Here's how the part is built. I have some questions about the finished solid (model axes, mm). Face numbers are marked on the shaded views. Coordinates: 2 decimals unless noted, no trailing zeros. Write each loop counter-clockwise with the first axis right and the second up, starting at its lowest first coordinate (ties: lowest second). Pieces come first, ordered by that corner, then holes.
(1) Thinking about a two-plate mould opening in Z: for the marked faces 1 and 2, which applies, released by +Z, released by -Z, zero draft, split by the parting line, or undercut?
(2) For pin 1 Ø1.5 at (x, z) = (239, -0.5) entering from +Y, with a flat end and sliding along its axis, tell me the tip position at first contact or that it passes through.
(3) Imagine slicing it at A-A, the plane x = 247. List the corners of the cut face in (y, z) for me, plus the area to 3 significant figures.
(4) Imagine slicing it at C-C, the plane x = 222. List the corners of the cut face in (y, z) for me.
(5) Imagine slicing it at B-B, the plane y = 166.5. List the corners of the cut face in (x, z) for me, plus the area to 3 significant figures.
(6) Please list where these lines run through material, in increasing order: probe 1 along X at (y, z) = (191, -0.75); probe 2 along X at (y, z) = (187, -0.75); probe 3 along X at (y, z) = (167, -3.8).
(7) Imagine slicing it at D-D, the plane z = -2.7. State how many separate pieces and enclosed holes the cut face has, plus the area to 3 significant figures.
Autodesk Inventor part; units mm, degrees
ref_plane "YZ Plane" through (0, 0, 0) normal (1, 0, 0) x (0, 1, 0)
ref_plane "XZ Plane" through (0, 0, 0) normal (0, 1, 0) x (-1, 0, 0)
ref_plane "XY Plane" through (0, 0, 0) normal (0, 0, 1) x (1, 0, 0)
sketch "Sketch2" plane through (0, 0, 0) normal (0, 0, 1) x (1, 0, 0)
  line L0 (0, 0) -> (264.075, 76.1785) construction
  circle A0 centre (264.075, 76.1785) radius 3.2512
  line L1 (0, 0) -> (41.9951, 204.3053) construction
  circle A1 centre (41.9951, 204.3053) radius 3.2512
  line L2 (0, 0) -> (97.7, 279.7575) construction
  circle A2 centre (97.7, 279.7575) radius 3.2512
  line L3 (0, 0) -> (70.949, 72.7241) construction
  circle A3 centre (70.949, 72.7241) radius 3.2512
  circle A4 centre (0, 0) radius 142.24 construction
  circle A5 centre (124.1608, 127.2672) radius 35.56 construction
  circle A6 centre (124.1608, 127.2672) radius 30 construction
  circle A7 centre (97.7, 279.7575) radius 6.35 construction
  circle A8 centre (41.9951, 204.3053) radius 6.35 construction
  circle A9 centre (70.949, 72.7241) radius 6.35 construction
  circle A10 centre (264.075, 76.1785) radius 6.35 construction
  line L4 (102.6169, 283.7758) -> (268.9919, 80.1968)
  line L5 (71.0626, 66.3751) -> (264.1886, 69.8295)
  line L6 (64.7474, 71.3595) -> (35.7934, 202.9407)
  line L7 (36.8865, 208.0769) -> (92.5914, 283.5291)
  arc A11 (36.8865, 208.0769) -> (35.7934, 202.9407) centre (41.9951, 204.3053) ccw
  arc A12 (102.6169, 283.7758) -> (92.5914, 283.5291) centre (97.7, 279.7575) ccw
  arc A13 (264.1886, 69.8295) -> (268.9919, 80.1968) centre (264.075, 76.1785) ccw
  arc A14 (64.7474, 71.3595) -> (71.0626, 66.3751) centre (70.949, 72.7241) ccw
  circle A15 centre (124.1608, 127.2672) radius 25.4 construction
  circle A16 centre (141.898, 145.4482) radius 2.794
  circle A17 centre (123.847, 152.6653) radius 2.794
  circle A18 centre (105.9798, 145.0045) radius 2.794
  circle A19 centre (98.7627, 126.9534) radius 2.794
  circle A20 centre (106.4235, 109.0862) radius 2.794
  circle A21 centre (124.4746, 101.8691) radius 2.794
  circle A22 centre (142.3418, 109.5299) radius 2.794
  circle A23 centre (149.5588, 127.581) radius 2.794
  circle A24 centre (124.1608, 127.2672) radius 9.652
  dimension "d84" = 50.8
  dimension "d63" = 6.5024
  dimension "d64" = 274.8432
  dimension "d65" = 76.1785
  dimension "d66" = 208.5767
  dimension "d67" = 6.5024
  dimension "d68" = 204.3053
  dimension "d69" = 6.5024
  dimension "d70" = 296.3268
  dimension "d71" = 279.7575
  dimension "d72" = 101.6
  dimension "d73" = 6.5024
  dimension "d74" = 72.7241
  dimension "d75" = 284.48
  dimension "d76" = 71.12
  dimension "d77" = 60
  dimension "d78" = 12.7
  dimension "d79" = 12.7
  dimension "d80" = 12.7
  dimension "d81" = 12.7
  dimension "d85" = 5.588
  dimension "d88" = 360
  dimension "d142" = 19.304
extrude "Extrusion5" add sketch "Sketch2" against normal blind 4.7625
sketch "Sketch4" plane through (0, 0, 0) normal (0, 0, 1) x (1, 0, 0)
  line L0 (35.7934, 202.9407) -> (64.7474, 71.3595) construction
  arc A0 (64.7474, 71.3595) -> (71.0626, 66.3751) centre (70.949, 72.7241) ccw construction
  line L1 (71.0626, 66.3751) -> (264.1886, 69.8295) construction
  arc A1 (264.1886, 69.8295) -> (268.9919, 80.1968) centre (264.075, 76.1785) ccw construction
  line L2 (268.9919, 80.1968) -> (102.6169, 283.7758) construction
  arc A2 (102.6169, 283.7758) -> (92.5914, 283.5291) centre (97.7, 279.7575) ccw construction
  line L3 (92.5914, 283.5291) -> (36.8865, 208.0769) construction
  arc A3 (36.8865, 208.0769) -> (35.7934, 202.9407) centre (41.9951, 204.3053) ccw construction
  circle A4 centre (97.7, 279.7575) radius 3.2512 construction
  circle A5 centre (98.7627, 126.9534) radius 2.794 construction
  circle A6 centre (124.1608, 127.2672) radius 9.652 construction
  circle A7 centre (149.5588, 127.581) radius 2.794 construction
  circle A8 centre (142.3418, 109.5299) radius 2.794 construction
  circle A9 centre (124.4746, 101.8691) radius 2.794 construction
  circle A10 centre (106.4235, 109.0862) radius 2.794 construction
  circle A11 centre (105.9798, 145.0045) radius 2.794 construction
  circle A12 centre (123.847, 152.6653) radius 2.794 construction
  circle A13 centre (141.898, 145.4482) radius 2.794 construction
  circle A14 centre (70.949, 72.7241) radius 3.2512 construction
  circle A15 centre (41.9951, 204.3053) radius 3.2512 construction
  circle A16 centre (264.075, 76.1785) radius 3.2512 construction
  circle A17 centre (41.9951, 204.3053) radius 9.6012 construction
  circle A18 centre (70.949, 72.7241) radius 9.6012 construction
  circle A19 centre (124.1608, 127.2672) radius 16.002 construction
  circle A20 centre (98.7627, 126.9534) radius 9.144 construction
  circle A21 centre (105.9798, 145.0045) radius 9.144 construction
  circle A22 centre (106.4235, 109.0862) radius 9.144 construction
  circle A23 centre (124.4746, 101.8691) radius 9.144 construction
  circle A24 centre (142.3418, 109.5299) radius 9.144 construction
  circle A25 centre (149.5588, 127.581) radius 9.144 construction
  circle A26 centre (141.898, 145.4482) radius 9.144 construction
  circle A27 centre (123.847, 152.6653) radius 9.144 construction
  circle A28 centre (97.7, 279.7575) radius 9.6012 construction
  circle A29 centre (264.075, 76.1785) radius 9.6012 construction
  line L4 (97.7, 279.7575) -> (264.075, 76.1785) construction
  line L5 (264.075, 76.1785) -> (70.949, 72.7241) construction
  line L6 (70.949, 72.7241) -> (41.9951, 204.3053) construction
  line L7 (41.9951, 204.3053) -> (97.7, 279.7575) construction
  line L8 (97.7, 279.7575) -> (123.847, 152.6653) construction
  line L9 (123.847, 152.6653) -> (105.9798, 145.0045) construction
  line L10 (105.9798, 145.0045) -> (41.9951, 204.3053) construction
  line L11 (115.7983, 160.2758) -> (96.5081, 254.0391)
  line L12 (87.9892, 255.9131) -> (53.0131, 208.5381)
  line L13 (53.6088, 202.1995) -> (104.1609, 155.348)
  line L14 (111.1656, 154.137) -> (113.0028, 154.9247)
  arc A30 (96.5081, 254.0391) -> (87.9892, 255.9131) centre (91.8309, 253.0769) ccw
  arc A31 (53.0131, 208.5381) -> (53.6088, 202.1995) centre (56.8548, 205.7018) ccw
  arc A32 (108.1503, 153.8871) -> (106.9173, 154.1003) centre (105.9798, 145.0045) ccw
  arc A33 (116.3014, 157.8302) -> (115.2975, 155.9086) centre (123.847, 152.6653) ccw construction
  arc A34 (113.0028, 154.9247) -> (115.7983, 160.2758) centre (111.121, 159.3135) ccw
  arc A35 (108.1503, 153.8871) -> (111.1656, 154.137) centre (109.2838, 158.5258) ccw
  arc A36 (104.1609, 155.348) -> (106.9173, 154.1003) centre (107.4069, 158.8503) ccw
  line L15 (148.9783, 151.2346) -> (181.2088, 177.5749) construction
  line L16 (132.3375, 149.2706) -> (133.4075, 148.8428) construction
  line L17 (133.9716, 155.456) -> (136.4882, 154.4499)
  line L18 (144.3569, 155.6585) -> (173.493, 179.47)
  line L19 (128.3811, 162.1383) -> (110.277, 250.1367)
  arc A37 (131.6628, 157.4114) -> (129.8982, 159.5206) centre (123.847, 152.6653) ccw
  arc A38 (141.5282, 154.5847) -> (139.5087, 154.2745) centre (141.898, 145.4482) ccw
  line L20 (174.1687, 186.1893) -> (118.6517, 254.1207)
  arc A39 (118.6517, 254.1207) -> (110.277, 250.1367) centre (114.9542, 251.0989) ccw
  arc A40 (173.493, 179.47) -> (174.1687, 186.1893) centre (170.4712, 183.1675) ccw
  arc A41 (141.5282, 154.5847) -> (144.3569, 155.6585) centre (141.3351, 159.356) ccw
  arc A42 (136.4882, 154.4499) -> (139.5087, 154.2745) centre (138.2609, 158.8838) ccw
  arc A43 (131.6628, 157.4114) -> (133.9716, 155.456) centre (135.7444, 159.89) ccw
  arc A44 (128.3811, 162.1383) -> (129.8982, 159.5206) centre (133.0583, 163.1006) ccw
  line L21 (157.901, 123.8365) -> (255.3158, 80.1103) construction
  line L22 (145.5014, 137.0441) -> (145.9555, 135.9851) construction
  line L23 (152.4019, 145.8317) -> (185.2271, 172.6581)
  line L24 (151.0349, 140.2524) -> (152.0986, 137.7715)
  line L25 (159.7907, 129.9486) -> (255.091, 87.1715)
  line L26 (185.2271, 172.6581) -> (255.091, 87.1715)
  arc A45 (150.327, 141.9034) -> (151.011, 144.6949) centre (141.898, 145.4482) ccw construction
  arc A46 (157.5651, 131.9983) -> (154.1105, 135.5117) centre (149.5588, 127.581) ccw
  arc A47 (152.0986, 137.7715) -> (154.1105, 135.5117) centre (156.4874, 139.6532) ccw
  arc A48 (157.5651, 131.9983) -> (159.7907, 129.9486) centre (161.7462, 134.3051) ccw
  arc A49 (152.4019, 145.8317) -> (151.0349, 140.2524) centre (155.4237, 142.1342) ccw
  line L27 (77.6537, 79.5965) -> (100.0381, 102.541) construction
  line L28 (114.9141, 105.6915) -> (115.984, 105.2638) construction
  line L29 (133.9377, 105.9266) -> (132.8787, 105.4725) construction
  line L30 (146.1642, 119.0905) -> (145.7364, 118.0205) construction
  line L31 (88.0917, 81.2024) -> (105.1273, 98.6642)
  line L32 (111.8334, 100.0845) -> (114.3499, 99.0784)
  line L33 (137.156, 100.3974) -> (134.6651, 99.3294)
  line L34 (151.1496, 114.4549) -> (151.0318, 114.1602)
  line L35 (157.539, 117.0386) -> (229.6718, 84.6606)
  line L36 (227.8018, 75.5297) -> (91.5952, 73.0934)
  arc A50 (80.5487, 72.8958) -> (80.5232, 73.4445) centre (70.949, 72.7241) ccw
  arc A51 (107.8174, 100.049) -> (108.8129, 100.2599) centre (106.4235, 109.0862) ccw
  arc A52 (116.6588, 97.123) -> (132.4053, 97.3175) centre (124.4746, 101.8691) ccw
  arc A53 (140.1713, 100.6473) -> (150.9905, 112.4987) centre (142.3418, 109.5299) ccw
  arc A54 (157.539, 117.0386) -> (151.1496, 114.4549) centre (155.5835, 112.6821) ccw
  circle A55 centre (153.2487, 113.2738) radius 2.3876 construction
  arc A56 (151.0318, 114.1602) -> (150.9905, 112.4987) centre (153.2487, 113.2738) ccw
  arc A57 (140.1713, 100.6473) -> (137.156, 100.3974) centre (139.0377, 96.0086) ccw
  arc A58 (134.6651, 99.3294) -> (132.4053, 97.3175) centre (136.5468, 94.9406) ccw
  arc A59 (116.6588, 97.123) -> (114.3499, 99.0784) centre (112.5772, 94.6444) ccw
  arc A60 (111.8334, 100.0845) -> (108.8129, 100.2599) centre (110.0607, 95.6506) ccw
  arc A61 (107.8174, 100.049) -> (105.1273, 98.6642) centre (108.5454, 95.3296) ccw
  arc A62 (88.0917, 81.2024) -> (91.5952, 73.0934) centre (91.5098, 77.8678) ccw
  arc A63 (227.8018, 75.5297) -> (229.6718, 84.6606) centre (227.7164, 80.3041) ccw
  line L37 (102.5851, 136.5139) -> (102.1573, 135.4439) construction
  line L38 (102.3661, 118.5493) -> (102.8202, 117.4902) construction
  line L39 (96.223, 116.7629) -> (97.291, 114.272)
  line L40 (96.9781, 139.5946) -> (95.972, 137.078)
  line L41 (75.4962, 86.4783) -> (96.0368, 107.5329)
  arc A64 (97.5409, 111.2567) -> (97.3547, 110.2564) centre (106.4235, 109.0862) ccw
  arc A65 (94.0166, 134.7692) -> (94.2111, 119.0227) centre (98.7627, 126.9534) ccw
  line L42 (95.5281, 146.0333) -> (55.5759, 183.0608)
  line L43 (47.6663, 178.5323) -> (67.4145, 88.7867)
  arc A66 (67.4145, 88.7867) -> (75.4962, 86.4783) centre (72.0781, 89.8129) ccw
  arc A67 (96.0368, 107.5329) -> (97.3547, 110.2564) centre (92.6188, 110.8675) ccw
  arc A68 (97.5409, 111.2567) -> (97.291, 114.272) centre (92.9022, 112.3902) ccw
  arc A69 (96.223, 116.7629) -> (94.2111, 119.0227) centre (91.8342, 114.8812) ccw
  arc A70 (94.0166, 134.7692) -> (95.972, 137.078) centre (91.538, 138.8508) ccw
  arc A71 (96.9813, 143.3795) -> (97.1534, 142.6151) centre (105.9798, 145.0045) ccw
  arc A72 (96.9813, 143.3795) -> (95.5281, 146.0333) centre (92.2821, 142.5309) ccw
  arc A73 (96.9781, 139.5946) -> (97.1534, 142.6151) centre (92.5442, 141.3673) ccw
  arc A74 (55.5759, 183.0608) -> (47.6663, 178.5323) centre (52.33, 179.5585) ccw
  point P0 (0, 0)
  point P1 (105.4705, 154.1343)
  point P2 (109.5245, 153.4334)
  point P3 (132.3137, 156.1189)
  point P4 (138.1461, 153.787)
  point P5 (142.9743, 154.5287)
  point P6 (177.1904, 182.4918)
  point P7 (128.7409, 160.3894)
  point P8 (106.3641, 269.156)
  point P9 (152.8022, 136.1304)
  point P10 (158.1618, 130.6798)
  point P11 (106.3742, 99.9423)
  point P12 (110.1755, 100.7474)
  point P13 (116.0079, 98.4155)
  point P14 (138.797, 101.101)
  point P15 (133.024, 98.6258)
  point P16 (249.1627, 75.9118)
  point P17 (95.5193, 118.4039)
  point P18 (97.9946, 112.631)
  point P19 (97.641, 141.2525)
  point P20 (95.3091, 135.4201)
  point P21 (71.4326, 82.3131)
  point P22 (97.2837, 108.8109)
  point P23 (96.8376, 144.8195)
  point P24 (44.3882, 193.4295)
  point P25 (68.8857, 82.101)
  dimension "d145" = 6.35
  dimension "d146" = 6.35
  dimension "d147" = 6.35
  dimension "d148" = 6.35
  dimension "d149" = 6.35
  dimension "d150" = 6.35
  dimension "d151" = 6.35
  dimension "d152" = 6.35
  dimension "d153" = 6.35
  dimension "d154" = 6.35
  dimension "d155" = 6.35
  dimension "d156" = 6.35
  dimension "d157" = 6.35
  dimension "d158" = 6.35
  dimension "d159" = 6.35
  dimension "d160" = 4.7752
  dimension "d161" = 4.7752
  dimension "d162" = 6.35
  dimension "d163" = 6.35
  dimension "d164" = 6.35
  dimension "d165" = 4.7752
  dimension "d166" = 6.35
  dimension "d167" = 6.35
  dimension "d168" = 6.35
  dimension "d169" = 4.7752
  dimension "d170" = 6.35
  dimension "d171" = 6.35
  dimension "d172" = 6.35
  dimension "d173" = 6.35
  dimension "d174" = 6.35
  dimension "d175" = 4.7752
  dimension "d176" = 4.7752
  dimension "d177" = 4.7752
  dimension "d178" = 4.7752
  dimension "d179" = 6.35
  dimension "d180" = 6.35
  dimension "d181" = 6.35
  dimension "d182" = 6.35
  dimension "d183" = 4.7752
  dimension "d184" = 4.7752
  dimension "d185" = 4.7752
extrude "Extrusion6" cut sketch "Sketch4" against normal blind 4.7625
properties part number "SHOT_1_015_PivotCover" material "Aluminum 6061"
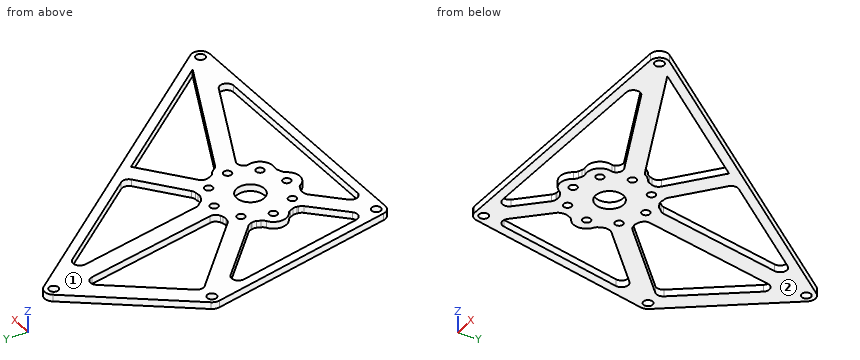
Recorded:
1. face 1: released by +Z
1. face 2: released by -Z
2. pin 1: stops at y = 117.81
3. outline: (69.52, -4.76) - (90.8, -4.76) - (90.8, 0) - (69.52, 0) - close; (97.07, -4.76) - (107.11, -4.76) - (107.11, 0) - (97.07, 0) - close
3. area: 149 mm2
4. outline: (69.07, -4.76) - (75.43, -4.76) - (75.43, 0) - (69.07, 0) - close; (88.1, -4.76) - (102.02, -4.76) - (102.02, 0) - (88.1, 0) - close; (127.66, -4.76) - (137.7, -4.76) - (137.7, 0) - (127.66, 0) - close
5. outline: (43.81, -4.76) - (50.31, -4.76) - (50.31, 0) - (43.81, 0) - close; (73.44, -4.76) - (92.13, -4.76) - (92.13, 0) - (73.44, 0) - close; (114.52, -4.76) - (127.48, -4.76) - (127.48, 0) - (114.52, 0) - close; (157.62, -4.76) - (177.69, -4.76) - (177.69, 0) - (157.62, 0) - close; (190.26, -4.76) - (198.46, -4.76) - (198.46, 0) - (190.26, 0) - close
5. area: 316 mm2
6. probe 1: x = 38.42 to 65.69, 109.48 to 122.44, 170.24 to 178.44
6. probe 2: x = 39.3 to 70.01, 110.3 to 123.27, 173.51 to 181.71
6. probe 3: x = 43.7 to 50.2, 72.91 to 91.59, 114.41 to 127.38, 158.23 to 178.3, 189.85 to 198.05
7. separate pieces: 1
7. enclosed holes: 18
7. area: 12,800 mm2
